Geometry: final body of the model. Coordinates: model frame, mm. A direction names the side the tool comes from. Round coordinates to 2 decimals unless told otherwise and drop trailing zeros. Loops run counter-clockwise (first coordinate to the right, second up) from the corner with the lowest first, then second, coordinate; pieces in that order, holes last. Notation, with made-up numbers: M 47,15 L 98,15 A22 ccw 98,44 Z; hole C -35.5,73.5 d3. An arc over 180 degrees is marked long. Write each question's results on one line, items separated by ' | '.
Autodesk Inventor part; units mm, degrees
ref_plane "YZ Plane" through (0, 0, 0) normal (1, 0, 0) x (0, 1, 0)
ref_plane "XZ Plane" through (0, 0, 0) normal (0, 1, 0) x (-1, 0, 0)
ref_plane "XY Plane" through (0, 0, 0) normal (0, 0, 1) x (1, 0, 0)
sketch "Boceto1" plane through (0, 0, 0) normal (0, 1, 0) x (-1, 0, 0)
  line L0 (-10, -9) -> (10, -9)
  line L1 (10, -9) -> (10, 9)
  line L2 (10, 9) -> (-10, 9)
  line L3 (-10, 9) -> (-10, -9)
  line L4 (-10, -9) -> (10, 9) construction
  line L5 (10, -9) -> (-10, 9) construction
  line L6 (-15, -15) -> (15, -15)
  line L7 (15, -15) -> (15, 15)
  line L8 (15, 15) -> (-15, 15)
  line L9 (-15, 15) -> (-15, -15)
  line L10 (-15, -15) -> (15, 15) construction
  line L11 (15, -15) -> (-15, 15) construction
  point P0 (0, 0)
  dimension "d0" = 20
  dimension "d1" = 18
  dimension "d2" = 30
  dimension "d3" = 30
extrude "Extrusión1" add sketch "Boceto1" along normal blind 18
sketch "Boceto2" plane through (0, 18, 0) normal (0, 1, 0) x (1, 0, 0)
  line L0 (10, 12) -> (-10, 12)
  line L1 (-10, 12) -> (-10, -12)
  line L2 (-10, -12) -> (10, -12)
  line L3 (10, -12) -> (10, 12)
  line L4 (10, 12) -> (-10, -12) construction
  line L5 (-10, 12) -> (10, -12) construction
  line L6 (-15, 15) -> (-15, -15)
  line L7 (-15, -15) -> (15, -15)
  line L8 (15, -15) -> (15, 15)
  line L9 (15, 15) -> (-15, 15)
  line L10 (10, 9) -> (10, -9)
  line L11 (10, -9) -> (-10, -9)
  line L12 (-10, -9) -> (-10, 9)
  line L13 (-10, 9) -> (10, 9)
  point P0 (0, 0)
  dimension "d6" = 20
  dimension "d7" = 24
extrude "Extrusión2" add sketch "Boceto2" along normal blind 15
sketch "Boceto4" plane through (15, 0, 15) normal (1, 0, 0) x (0, 0, -1)
  line L0 (30, 0) -> (30, 33)
  line L1 (0, 0) -> (0, 33)
  line L2 (30, 0) -> (0, 0)
  line L3 (0, 0) -> (0, 12)
  line L4 (0, 12) -> (30, 12)
  line L5 (30, 12) -> (30, 0)
  point P0 (15, 0)
  dimension "d13" = 12
extrude "Extrusión4" add sketch "Boceto4" along normal blind 25
sketch "Boceto5" plane through (15, 12, 15) normal (0, 1, 0) x (1, 0, 0)
  circle A0 centre (18, 7) radius 2.35
  circle A1 centre (18, 23) radius 2.35
  line L0 (25, 30) -> (25, 0)
  line L1 (0, 0) -> (25, 0)
  line L2 (0, 30) -> (25, 30)
  point P0 (-15, 15)
  dimension "d16" = 4.7
  dimension "d17" = 4.7
  dimension "d18" = 7
  dimension "d19" = 7
  dimension "d20" = 7
  dimension "d21" = 7
extrude "Extrusión5" cut sketch "Boceto5" against normal through all
sketch "Boceto6" plane through (0, 33, 0) normal (0, 1, 0) x (1, 0, 0)
  line L0 (10, 9) -> (10, -9)
  line L1 (10, -2.5) -> (13, -2.5)
  line L2 (13, -2.5) -> (13, 2.5)
  line L3 (13, 2.5) -> (10, 2.5)
  line L4 (10, 2.5) -> (10, -2.5)
  point P0 (0, 0)
  point P1 (10, 0)
  dimension "d24" = 5
  dimension "d25" = 3
extrude "Extrusión6" cut sketch "Boceto6" against normal blind 5
sketch "Boceto7" plane through (15, 33, 15) normal (1, 0, 0) x (0, 0, -1)
  circle A0 centre (6.3, -9.5) radius 1.475
  circle A1 centre (23.7, -9.5) radius 1.475
  line L0 (30, -21) -> (0, -21)
  line L1 (0, -21) -> (0, 0)
  line L2 (30, -21) -> (30, 0)
  line L3 (6.3, -9.5) -> (23.7, -9.5)
  line L4 (0, -33) -> (30, -33)
  point P0 (15, -33)
  point P1 (15, -9.5)
  point P2 (15, -33)
  dimension "d28" = 2.95
  dimension "d30" = 11.5
  dimension "d32" = 11.5
  dimension "d34" = 17.4
extrude "Extrusión7" cut sketch "Boceto7" against normal blind 5
sketch "Boceto8" plane through (-15, 0, -15) normal (-1, 0, 0) x (0, 0, 1)
  line L0 (0, 33) -> (30, 33)
  line L1 (30, 12) -> (30, 33)
  line L2 (0, 33) -> (30, 33)
  line L3 (30, 33) -> (30, 18)
  line L4 (30, 18) -> (0, 18)
  line L5 (0, 18) -> (0, 33)
  point P0 (15, 0)
  dimension "d43" = 15
extrude "Extrusión8" cut sketch "Boceto8" against normal blind 2
sketch "Boceto9" plane through (40, 0, -15) normal (0, 0, -1) x (-1, 0, 0)
  line L0 (50, 33) -> (30, 33)
  line L1 (46, 33) -> (49, 33)
  line L2 (49, 33) -> (49, 0)
  line L3 (49, 0) -> (46, 0)
  line L4 (46, 0) -> (46, 33)
  line L5 (53, 18) -> (53, 33)
  point P0 (40, 0)
  dimension "d46" = 3
  dimension "d47" = 4
extrude "Extrusión9" add sketch "Boceto9" along normal blind 8
sketch "Boceto10" plane through (-9, 0, -15) normal (-1, 0, 0) x (0, 0, 1)
  line L0 (0, 33) -> (-8, 33)
  line L1 (0, 0) -> (-8, 0)
  line L2 (-8, 33) -> (-5, 33)
  line L3 (-5, 33) -> (-5, 0)
  line L4 (-5, 0) -> (-8, 0)
  line L5 (-8, 0) -> (-8, 33)
  point P0 (15, 0)
  point P1 (-8, 0)
  dimension "d50" = 3
extrude "Extrusión10" add sketch "Boceto10" along normal blind 16
sketch "Boceto11" plane through (40, 0, -23) normal (0, 0, -1) x (-1, 0, 0)
  circle A0 centre (57, 22) radius 1.475
  line L0 (46, 33) -> (65, 33)
  line L1 (46, 33) -> (46, 0)
  point P0 (40, 0)
  dimension "d53" = 2.95
  dimension "d54" = 11
  dimension "d55" = 11
extrude "Extrusión11" cut sketch "Boceto11" against normal up to surface (3 mm away)
properties part number "Soporte_motor"
1. Section A-A (z = -1). Output: boundary loops of the cut face in (x, y), then the cut area to 3 significant figures.
Answer key:
outline: M -15,0 L -10,0 L -10,33 L -13,33 L -13,18 L -15,18 Z; M 10,0 L 40,0 L 40,12 L 15,12 L 15,33 L 13,33 L 13,28 L 10,28 Z | area: 585 mm²
2. Ray query, probe 1 along X at (y, z) = (3, -3.5); probe 2 along X at (y, z) = (4.25, -8); probe 3 along X at (y, z) = (17, -8). Return the intervals inside material, ascending.
Answer key:
probe 1: x = -15 to -10, 10 to 40 | probe 2: x = -15 to -10, 10 to 30.65, 35.35 to 40 | probe 3: x = -15 to -10, 10 to 15
3. Section C-C (y = 10). Output: boundary loops of the cut face in (x, z).
Answer key:
outline: M -25,-23 L -6,-23 L -6,-15 L 40,-15 L 40,15 L -15,15 L -15,-15 L -9,-15 L -9,-20 L -25,-20 Z; hole M -10,-9 L 10,-9 L 10,9 L -10,9 Z; hole C 33,-8 d4.7; hole C 33,8 d4.7
4. Access query for faces 1 (the face through (12.54, 22.06, 9.02)), 2 (the face through (-11, 16, -15)), 3 (the face through (27, 12, 0)), 4 (the face through (11, 28, 0)), 5 (the face through (-6, 16, -19)). Directions: +Z, -Z, +X, -X, +Y, -Y. A direction counts if a zero-diameter tool reaches every point of the face in a straight line with its end or side. Return the directions, or none.
Answer key:
face 1: +X | face 2: -X, +Y, -Y | face 3: +Z, -Z, +X, +Y | face 4: +Y | face 5: -Z, +X, +Y, -Y
5. Section B-B (x = 33). Output: boundary loops of the cut face in (y, z).
Answer key:
outline: M 0,-15 L 12,-15 L 12,-10.35 L 0,-10.35 Z; M 0,-5.65 L 12,-5.65 L 12,5.65 L 0,5.65 Z; M 0,10.35 L 12,10.35 L 12,15 L 0,15 Z
6. Section D-D (x = 3). Output: boundary loops of the cut face in (y, z).
Answer key:
outline: M 0,-15 L 33,-15 L 33,-12 L 18,-12 L 18,-9 L 0,-9 Z; M 0,9 L 18,9 L 18,12 L 33,12 L 33,15 L 0,15 Z
7. Pin query (flat end, axial travel): P1, Ø16.5, axis at x = -2.5, y = 28, coming from the -Z side; P2, Ø10, axis at x = 18.5, y = 18, coming from the -Z side; P3, Ø3, axis at x = 33, z = -8, coming from the +Y side; P4, Ø12, axis at y = 19.5, z = 3.5, coming from the +X side. Return the tip coordinate at first contact, or that it passes through.
Answer key:
P1: stops at z = -23 | P2: stops at z = -15 | P3: passes through | P4: stops at x = 15
8. Draft query along X for faces 6 (the face through (10, 16, 0)), 7 (the face through (-10, 16, 0)), 8 (the face through (-1.9, 33, -12.4)), 9 (the face through (-13, 26, 0)). Return one class per face: pulls with the +X half, pulls with the -X half, needs draft (parallel to the pull), parting line crosses it, or undercut.
Answer key:
face 6: undercut | face 7: undercut | face 8: needs draft | face 9: pulls with the -X half
